The figure shows three views and two pictorial views of one solid part (mm, origin at its lowest corner). Answer the questions. A direction names the side the tool comes from. Coordinates: 2 decimals unless noted, no trailing zeros. Write each loop counter-clockwise with the first axis right and the second up, starting at its lowest first coordinate (ties: lowest second). Pieces come first, ordered by that corner, then holes.
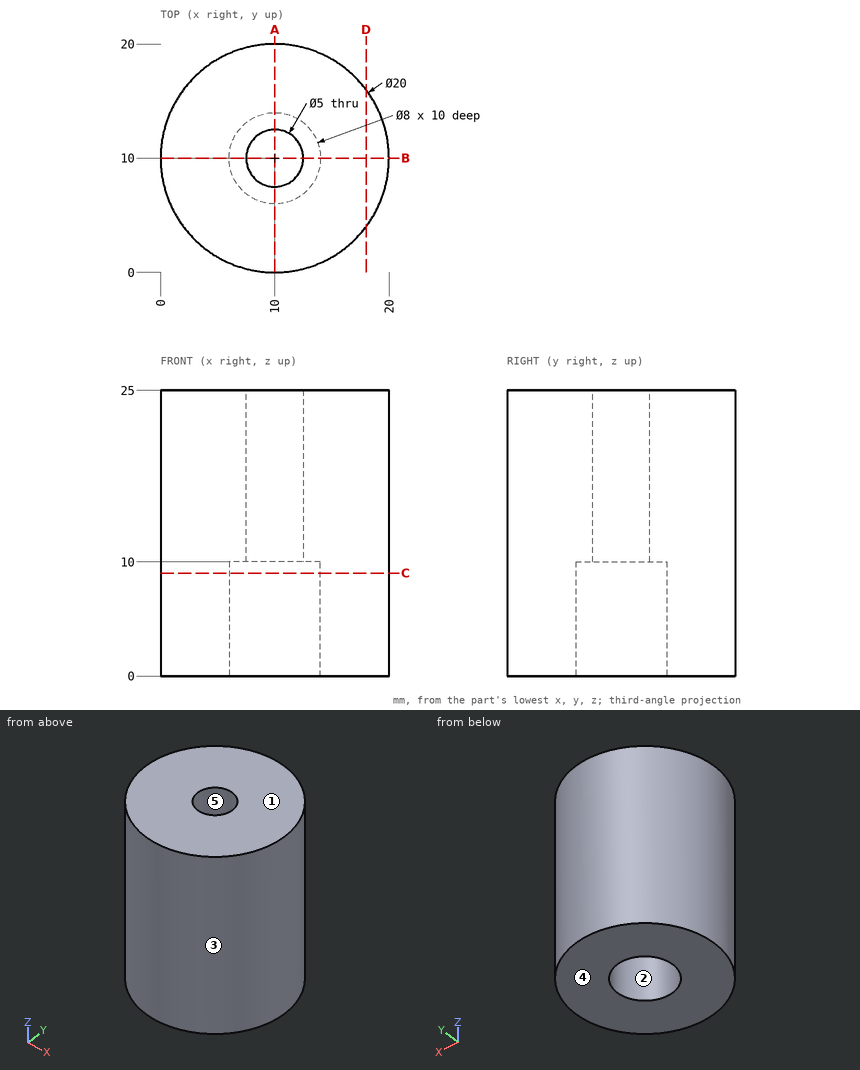
1. Section C-C on z = 9 is taken. Give the vertices of the cut face in (x, y).
Results found:
outline: circle Ø20 at (10, 10); hole circle Ø8 at (10, 10)
2. For a pull along Y with two mould halves and no side action, classify the marked faces 3, 4 and 5 as pulls with the +Y half, pulls with the -Y half, needs draft (parallel to the pull), parting line crosses it, or undercut.
Results found:
face 3: parting line crosses it
face 4: needs draft
face 5: undercut
3. Flat-ended cylindrical pins translate along their axes: P1, Ø12, axis at x = 17, y = 3, coming from the -Z side; P2, Ø3, axis at y = 6.5, z = 7, coming from the -X side; P3, Ø4.5, axis at x = 10, y = 10, coming from the -Z side; P4, Ø12, axis at x = 3.5, z = 13.5, coming from the +Y side. Find the tip coordinate at first contact, or state that the pin passes through.
Results found:
P1: stops at z = 0
P2: stops at x = 0.2
P3: passes through
P4: stops at y = 19.99
4. A tool of negligible diameter and unlimited length cuts with its end or side. For the marked faces 1 and 2, from which of +Z, -Z, +X, -X, +Y, -Y can it reach the whole face along a straight path? Write none if from no direction.
Results found:
face 1: +Z, +X, -X, +Y, -Y
face 2: -Z
5. Section D-D on x = 18 is taken. Give the vertices of the cut face in (y, z).
Results found:
outline: (4, 0) - (16, 0) - (16, 25) - (4, 25) - close
6. Find the intervals of material crossed by L1, parallel to Y at x = 10, z = 4; L2, parallel to Y at x = 10, z = 20.75; L3, parallel to X at y = 6.5, z = 7, in increasing order.
Results found:
L1: y = 0 to 6, 14 to 20
L2: y = 0 to 7.5, 12.5 to 20
L3: x = 0.63 to 8.06, 11.94 to 19.37
7. Section A-A on x = 10 is taken. Give the vertices of the cut face in (y, z).
Results found:
outline: (0, 0) - (6, 0) - (6, 10) - (7.5, 10) - (7.5, 25) - (0, 25) - close; (12.5, 10) - (14, 10) - (14, 0) - (20, 0) - (20, 25) - (12.5, 25) - close
